```python
from build123d import *

# Parameters (mm, degrees)
BOSS_EXTRUDE1_DEPTH             = 4.7625
TAP_DRILL_FOR_M6X1_0_TAP1_D     = 5
TAP_DRILL_FOR_M6X1_0_TAP1_DEPTH = 9.525


with BuildPart() as part:
    # Sketch1 → Boss-Extrude1 (new body, symmetric)
    with BuildSketch(Plane(origin=(0, 0, 0), x_dir=(1, 0, 0), z_dir=(0, 1, 0))):
        Polygon((-55, -1), (-55, 81), (55, 81), (55, -1), (115.5, -1), (115.5, -19), (-115.5, -19), (-115.5, -1), align=None)
    extrude(amount=BOSS_EXTRUDE1_DEPTH, both=True)

    # Tap Drill for M6x1.0 Tap1
    with Locations(Plane(origin=(0, 4.7625, 0), x_dir=(1, 0, 0), z_dir=(0, 1, 0))):
        with Locations((-45, 68.3), (45, 68.3), (-102.8, -10), (102.8, -10)):
            Hole(TAP_DRILL_FOR_M6X1_0_TAP1_D / 2, depth=TAP_DRILL_FOR_M6X1_0_TAP1_DEPTH)


solid = part.part
```
Input: part model. Units: mm. Frame: model coordinates. A direction names the side the tool comes from. Give positions to 0.01 mm unless a question says otherwise; leave off trailing zeros. Write each loop counter-clockwise with the first axis right and the second up, starting at its lowest first coordinate (ties: lowest second). Pieces come first, ordered by that corner, then holes. Notation, with made-up numbers: (67, 21) - (122, 21) arc R10 cw to (122, 39) - close; hole circle Ø2 at (-6, 84.25). An arc over 180 degrees is marked (long way). Write item = value, one per line. Start each with the question number.
1. Section query D-D, the plane z = 10. Output: boundary loops of the cut face in (x, y).
2. Ray query, L1, parallel to X at y = 1.25, z = 10; L2, parallel to X at y = -1.75, z = -68.3; L3, parallel to Z at x = -102.8, y = -2.25. Return the intervals inside material, ascending.
3. Section query A-A, the plane z = -68.3. Output: boundary loops of the cut face in (x, y), then the cut area to 4 significant figures.
4. Mould query, pull axis Z, two halves, no side actions, for faces 4 (the flat face through (115.5, 0, 10)), 5 (the flat face through (85, 0, 1)), 6 (the cylindrical face through (101.65, -0.07, 12.22)). Classes: released by +Z, released by -Z, zero draft, split by the parting line, or undercut.
5. First-contact query: pin 1 Ø1 at (y, z) = (0.5, -9.5) entering from +X; pin 2 Ø5 at (y, z) = (2, -23) entering from -X; pin 3 Ø2 at (x, y) = (89, 3) entering from -Z. Flat tips, straight axial feed; report the tip coordinate or a pass-through.
6. Access query for faces 1 (the cylindrical face through (-44.67, -0.07, -70.78)), 2 (the flat face through (-55, 0, -39)), 3 (the flat face through (55, 0, -41)). Directions: +Z, -Z, +X, -X, +Y, -Y. A direction counts if a zero-diameter tool reaches every point of the face in a straight line with its end or side. Return the directions, or none.
7. Section query B-B, the plane y = 2. Output: boundary loops of the cut face in (x, z), then the cut area to 3 significant figures.
8. Section query C-C, the plane x = -102.8. Output: boundary loops of the cut face in (y, z).
Check sheet entries:
q1.outline = (-115.5, -4.76) - (-105.3, -4.76) - (-105.3, 4.76) - (-115.5, 4.76) - close; (-100.3, -4.76) - (100.3, -4.76) - (100.3, 4.76) - (-100.3, 4.76) - close; (105.3, -4.76) - (115.5, -4.76) - (115.5, 4.76) - (105.3, 4.76) - close
q2.L1 = -115.5 to -105.3, -100.3 to 100.3, 105.3 to 115.5
q2.L2 = -55 to -47.5, -42.5 to 42.5, 47.5 to 55
q2.L3 = 1 to 7.5, 12.5 to 19
q3.outline = (-55, -4.76) - (-47.5, -4.76) - (-47.5, 4.76) - (-55, 4.76) - close; (-42.5, -4.76) - (42.5, -4.76) - (42.5, 4.76) - (-42.5, 4.76) - close; (47.5, -4.76) - (55, -4.76) - (55, 4.76) - (47.5, 4.76) - close
q3.area = 952.5 mm2
q4.face_4 = zero draft
q4.face_5 = released by -Z
q4.face_6 = undercut
q5.pin_1 = 55
q5.pin_2 = -55
q5.pin_3 = 1
q6.face_1 = +Y, -Y
q6.face_2 = -Z, -X, +Y, -Y
q6.face_3 = -Z, +X, +Y, -Y
q7.outline = (-115.5, 1) - (-55, 1) - (-55, -81) - (55, -81) - (55, 1) - (115.5, 1) - (115.5, 19) - (-115.5, 19) - close; hole circle Ø5 at (-102.8, 10); hole circle Ø5 at (-45, -68.3); hole circle Ø5 at (45, -68.3); hole circle Ø5 at (102.8, 10)
q7.area = 13,100 mm2
q8.outline = (-4.76, 1) - (4.76, 1) - (4.76, 7.5) - (-4.76, 7.5) - close; (-4.76, 12.5) - (4.76, 12.5) - (4.76, 19) - (-4.76, 19) - close
